Can you work these out from the drawing? Everything is in mm from the part's minimum corner. A direction names the side the tool comes from. Give positions to 0.01 mm unless a question says otherwise; leave off trailing zeros. Order: outer loops, then holes, each group sorted by start corner. A loop starts at its lowest first (then second) coordinate and runs counter-clockwise, first axis right, second up. Notation, with made-up numbers: (-33.5, -15) -> (-29.5, -15) arc R23 ccw to (-29.5, 20) -> close; hole circle Ø11 at (40, 64). An arc over 180 degrees is marked (long way). Answer as CSV lines item,"result". Start each with the question number.
(1) I need wall thicknesses on L1, parallel to Z at x = 2.75, y = 4.15; L2, parallel to X at y = 1.5, z = 1; L3, parallel to X at y = 2.35, z = 4.5. Which ranges of each line are inside material? Lowest first, please.
(2) Will these pins go through, and if not, where does the flat tip stop? pin 1 Ø2 at (y, z) = (0.5, 4) entering from +X; pin 2 Ø2 at (y, z) = (2.5, 5.5) entering from +X; pin 3 Ø1 at (y, z) = (1, 4) entering from -X.
(3) I want a section at D-D (z = 5.25). Please give me the cut outline in (x, y), plus the area to 3 significant figures.
(4) I want a section at A-A (y = 2.25). Please give me the cut outline in (x, z).
(5) On a 3-axis mill with a long thin cutter (end or side, diameter ignored), from which of +Z, -Z, +X, -X, +Y, -Y can I reach the whole of each face in a straight line? I mean the marked faces 1 and 2. Say none if no direction works.
(6) I want a section at C-C (z = 2). Please give me the cut outline in (x, y).
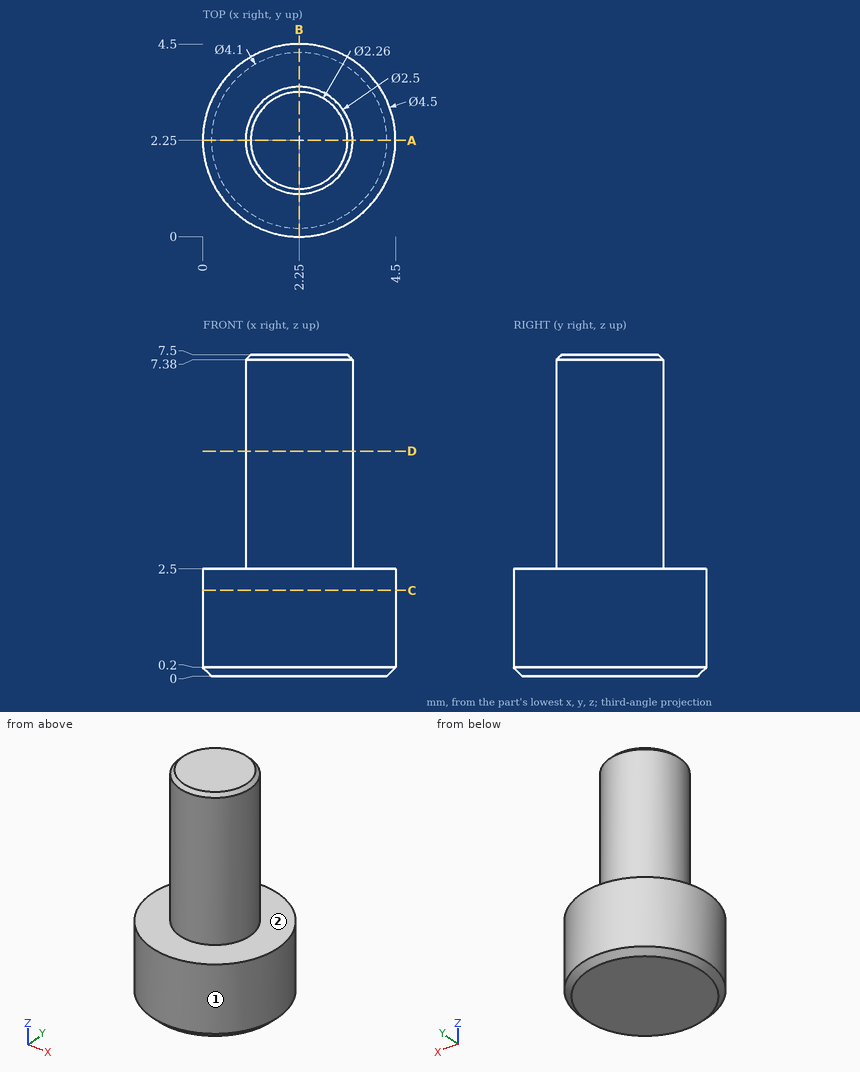
Final values:
1,L1,"0 to 2.5"
1,L2,"0.13 to 4.37"
1,L3,"1 to 3.5"
2,pin 1,"x = 3.25"
2,pin 2,"x = 3.5"
2,pin 3,"x = 1.25"
3,outline,"circle Ø2.5 at (2.25, 2.25)"
3,area,"4.91 mm²"
4,outline,"(0, 0.2) -> (0.2, 0) -> (4.3, 0) -> (4.5, 0.2) -> (4.5, 2.5) -> (3.5, 2.5) -> (3.5, 7.38) -> (3.38, 7.5) -> (1.12, 7.5) -> (1, 7.38) -> (1, 2.5) -> (0, 2.5) -> close"
5,face 1,"+Z, -Z"
5,face 2,"+Z"
6,outline,"circle Ø4.5 at (2.25, 2.25)"
